Study the drawing (mm; zero at the part's minimum x, y, z) and answer. A direction names the side the tool comes from. Give positions to 0.01 mm unless a question says otherwise; leave off trailing zeros. Loops run counter-clockwise (first coordinate to the right, second up) from the corner with the lowest first, then second, coordinate; pieces in that order, holes last. Notation, with made-up numbers: M -24,12 L 28,12 A16 ccw 28,25 Z; hole C 28.5,-24.75 d1. An arc over 180 degrees is marked long. Use one line per item in the form item = value. Start each with the question number.
1. Straight lines are drawn through the part: line 1 (Z direction, x = 6.25, y = 5.5); line 2 (Z direction, x = 2.5, y = 17.25); line 3 (X direction, y = 20.4, z = 11). For each, find the intervals that lie inside material, in ascending order. Write a range as from..to.
2. Each of these flat-tipped pins is pushed along its axis until it touches: pin 1 Ø2.5 at (x, z) = (17.55, 6.4) entering from +Y; pin 2 Ø0.9 at (x, y) = (19.5, 9.5) entering from +Z; pin 3 Ø4 at (x, z) = (13, 13) entering from -Y; pin 4 Ø2 at (x, y) = (14, 17.5) entering from -Z. Where does it stop, or does it pass through?
3. The part is cut by section D-D (x = 13.5). Write down the section's boundary in (y, z).
4. For the marked faces 5, 6, 7, 8 and 9, determine the directions among +Z, -Z, +X, -X, +Y, -Y from which every point of the face is accessible in a straight line to the end or side of a thin tool.
5. The part is cut by section A-A (z = 11). Write down the section's boundary in (x, y).
6. The part is cut by section C-C (y = 7.5). Write down the section's boundary in (x, z).
7. The mould has two halves that part along Z. Classify the marked faces 1, 2, 3 and 4: released by +Z, released by -Z, zero draft, split by the parting line, or undercut.
8. The part is cut by section B-B (y = 2.25). Write down the section's boundary in (x, z), and give its area (3 significant figures).
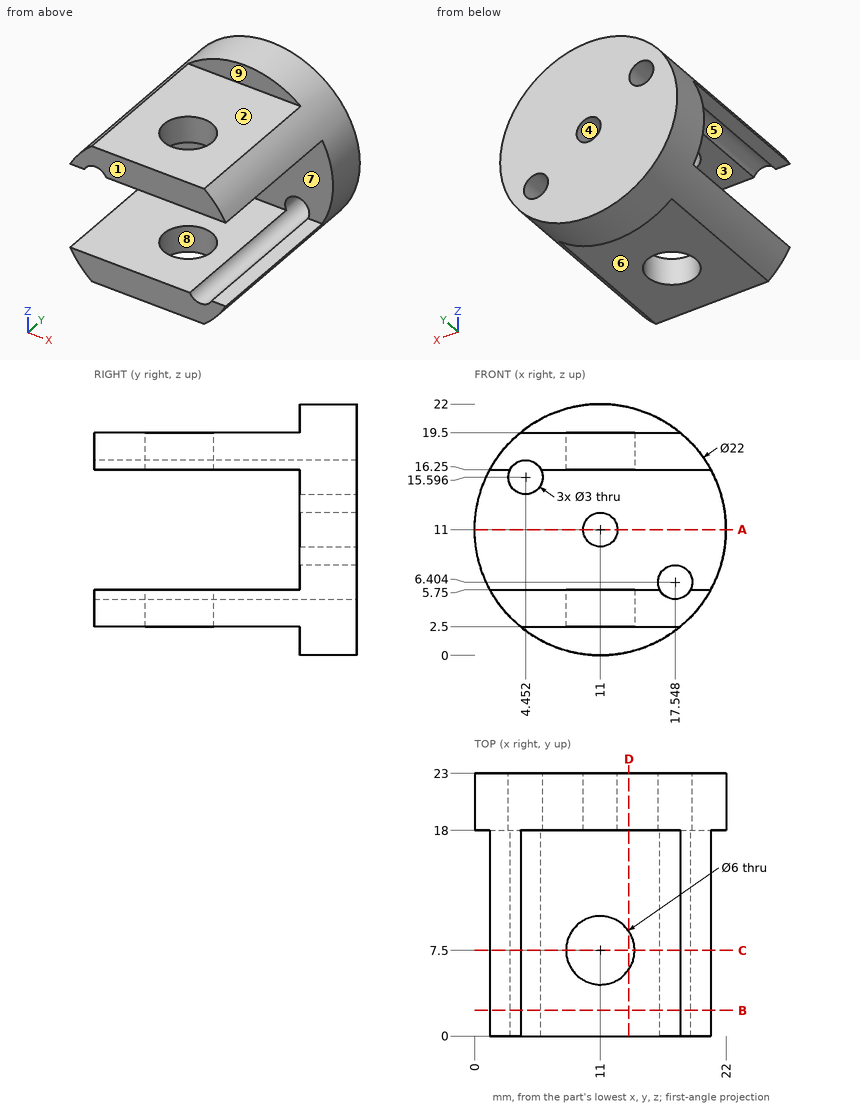
Derived:
q1.line_1 = 2.5..5.75, 16.25..19.5
q1.line_2 = 4.02..5.75, 16.25..17.98
q1.line_3 = 0..9.5, 12.5..22
q2.pin_1 = through
q2.pin_2 = 18.5
q2.pin_3 = 18
q2.pin_4 = 0.21
q3.outline = M 0,2.5 L 5.84,2.5 L 5.84,5.75 L 0,5.75 Z; M 0,16.25 L 5.84,16.25 L 5.84,19.5 L 0,19.5 Z; M 9.16,2.5 L 18,2.5 L 18,0.29 L 23,0.29 L 23,21.71 L 18,21.71 L 18,19.5 L 9.16,19.5 L 9.16,16.25 L 18,16.25 L 18,5.75 L 9.16,5.75 Z
q4.face_5 = +Y, -Y
q4.face_6 = -Z, +X, -X, -Y
q4.face_7 = +X, -X, -Y
q4.face_8 = +Z, -Z
q4.face_9 = +Z, +X, -X, -Y
q5.outline = M 0,18 L 9.5,18 L 9.5,23 L 0,23 Z; M 12.5,18 L 22,18 L 22,23 L 12.5,23 Z
q6.outline = M 1.33,5.75 A11 ccw 4.02,2.5 L 8,2.5 L 8,5.75 Z; M 1.33,16.25 L 3.1,16.25 A1.5 cw 5.8,16.25 L 8,16.25 L 8,19.5 L 4.02,19.5 A11 ccw Z; M 14,2.5 L 17.98,2.5 A11 ccw 20.67,5.75 L 18.9,5.75 A1.5 cw 16.2,5.75 L 14,5.75 Z; M 14,16.25 L 20.67,16.25 A11 ccw 17.98,19.5 L 14,19.5 Z
q7.face_1 = zero draft
q7.face_2 = released by +Z
q7.face_3 = undercut
q7.face_4 = undercut
q8.outline = M 1.33,5.75 A11 ccw 4.02,2.5 L 17.98,2.5 A11 ccw 20.67,5.75 L 18.9,5.75 A1.5 cw 16.2,5.75 Z; M 1.33,16.25 L 3.1,16.25 A1.5 cw 5.8,16.25 L 20.67,16.25 A11 ccw 17.98,19.5 L 4.02,19.5 A11 ccw Z
q8.area = 107 mm2
